Could you check a few things on this drawing? It's one solid part, dimensions in mm from its lowest x, y, z. A direction names the side the tool comes from. Round coordinates to 2 decimals unless told otherwise and drop trailing zeros. Write each loop counter-clockwise with the first axis right and the second up, starting at its lowest first coordinate (ties: lowest second). Pieces come first, ordered by that corner, then holes. Notation, with made-up numbers: M 80,-17.5 L 101,-17.5 A21 ccw 101,18.5 Z; hole C 73,40.5 d2. An arc over 180 degrees is marked long. One line per item, written item: value. Start each with the question number.
(1) If I drill on L1, parallel to X at y = 4.5, z = 44.8; L2, parallel to Z at x = 131.2, y = 4.25; L3, parallel to X at y = 7.25, z = 42, over which ranges is the centre line in solid material (lowest first)?
(2) I'm going to push flat-ended pins straight in: pin 1 Ø4 at (y, z) = (4, 5.5) entering from -X; pin 2 Ø2.5 at (x, y) = (64.5, 5.5) entering from +Z; pin 3 Ø4 at (y, z) = (3.5, 46.5) entering from +X. Where does each tip first touch, or does it pass through?
(3) Which directions (+Z, -Z, +X, -X, +Y, -Y) give clear straight access to the entire face, cutting with the end or side of a thin tool? Please do the marked faces 1 and 2.
(4) I want a section at B-B on x = 105.5. Please give me the cut outline in (y, z).
(5) I want a section at A-A on z = 44.8. Please give me the cut outline in (x, y).
(6) I want a section at D-D on z = 20. Please give me the cut outline in (x, y).
(7) I want a section at C-C on x = 80. Please give me the cut outline in (y, z), and give its area (3 significant figures).
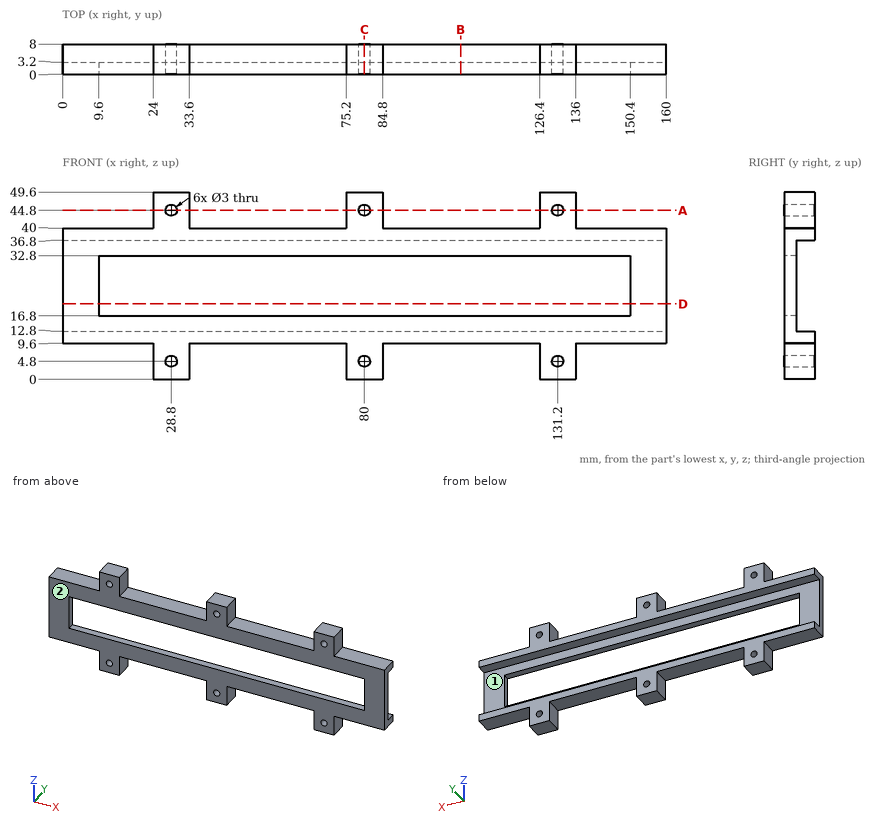
Found:
1. L1: x = 24 to 27.3, 30.3 to 33.6, 75.2 to 78.5, 81.5 to 84.8, 126.4 to 129.7, 132.7 to 136
1. L2: z = 0 to 3.3, 6.3 to 12.8, 36.8 to 43.3, 46.3 to 49.6
1. L3: x = 24 to 33.6, 75.2 to 84.8, 126.4 to 136
2. pin 1: stops at x = 24
2. pin 2: stops at z = 40
2. pin 3: stops at x = 136
3. face 1: +X, -X, +Y
3. face 2: +Z, -Z, +X, -X, -Y
4. outline: M 0,9.6 L 8,9.6 L 8,12.8 L 3.2,12.8 L 3.2,16.8 L 0,16.8 Z; M 0,32.8 L 3.2,32.8 L 3.2,36.8 L 8,36.8 L 8,40 L 0,40 Z
5. outline: M 24,0 L 27.3,0 L 27.3,8 L 24,8 Z; M 30.3,0 L 33.6,0 L 33.6,8 L 30.3,8 Z; M 75.2,0 L 78.5,0 L 78.5,8 L 75.2,8 Z; M 81.5,0 L 84.8,0 L 84.8,8 L 81.5,8 Z; M 126.4,0 L 129.7,0 L 129.7,8 L 126.4,8 Z; M 132.7,0 L 136,0 L 136,8 L 132.7,8 Z
6. outline: M 0,0 L 9.6,0 L 9.6,3.2 L 0,3.2 Z; M 150.4,0 L 160,0 L 160,3.2 L 150.4,3.2 Z
7. outline: M 0,0 L 8,0 L 8,3.3 L 0,3.3 Z; M 0,6.3 L 8,6.3 L 8,12.8 L 3.2,12.8 L 3.2,16.8 L 0,16.8 Z; M 0,32.8 L 3.2,32.8 L 3.2,36.8 L 8,36.8 L 8,43.3 L 0,43.3 Z; M 0,46.3 L 8,46.3 L 8,49.6 L 0,49.6 Z
7. area: 182 mm²
